Input: part model. Units: mm. Frame: model coordinates. A direction names the side the tool comes from. Give positions to 0.01 mm unless a question says otherwise; leave off trailing zeros. Loops run counter-clockwise (first coordinate to the right, second up) from the corner with the lowest first, then second, coordinate; pieces in that order, holes last. Notation, with made-up numbers: M 15.5,-32.75 L 25.5,-32.75 A8 cw 25.5,-19.75 Z; hole C 32,35.5 d1. An arc over 180 degrees is marked long. One line per item, written item: value. Start each with the question number.
(1) Ray query, line 1 along X through (y, z) = (2.5, 0.7); line 2 along X through (y, z) = (47.5, 2.05); line 3 along X through (y, z) = (31, 1.15). Return the intervals inside material, ascending. Write a range as from..to.
(2) Pull-direction query (X, two-part tool) for faces 6 (the flat face through (42, 30, 1)), 7 (the flat face through (50, 12, 1)), 8 (the flat face through (0, 13, 1)), 9 (the flat face through (25, 25, 3)); classes: released by +X, released by -X, zero draft, split by the parting line, or undercut.
(3) Section D-D on x = 38.5. Output: boundary loops of the cut face in (y, z).
(4) Section C-C on y = 2.5. Output: boundary loops of the cut face in (x, z).
(5) Section A-A on x = 25. Output: boundary loops of the cut face in (y, z).
(6) Access query for faces 1 (the flat face through (45, 37, 2)), 2 (the flat face through (25, 50, 1)), 3 (the flat face through (3, 25, 2)), 4 (the flat face through (38, 36.5, 1)), 5 (the flat face through (25, 25, 0)). Directions: +Z, -Z, +X, -X, +Y, -Y. A direction counts if a zero-diameter tool reaches every point of the face in a straight line with its end or side. Return the directions, or none.
(7) Pin query (flat end, axial travel): P1, Ø0.9, axis at x = 47, z = 1, coming from the +Y side; P2, Ø0.9, axis at y = 40, z = 1, coming from the -X side; P3, Ø1.5, axis at y = 29, z = 1.5, coming from the +X side. Return the tip coordinate at first contact, or that it passes through.
(8) Section B-B on z = 2.2. Output: boundary loops of the cut face in (x, y), plus the area to 3 significant figures.
Autodesk Inventor part; units mm, degrees
ref_plane "YZ Plane" through (0, 0, 0) normal (1, 0, 0) x (0, 1, 0)
ref_plane "XZ Plane" through (0, 0, 0) normal (0, 1, 0) x (-1, 0, 0)
ref_plane "XY Plane" through (0, 0, 0) normal (0, 0, 1) x (1, 0, 0)
sketch "Sketch1" plane through (0, 0, 0) normal (0, 0, 1) x (1, 0, 0)
  line L0 (0, 0) -> (50, 0)
  line L1 (50, 0) -> (50, 50)
  line L2 (50, 50) -> (0, 50)
  line L3 (0, 50) -> (0, 0)
  line L4 (25, 50) -> (25, 47.5)
  line L5 (0, 0) -> (5, 0)
  line L6 (5, 0) -> (5, 2.5)
  line L7 (50, 0) -> (45, 0)
  line L8 (45, 0) -> (45, 2.5)
  circle A0 centre (5, 2.5) radius 1.75
  circle A1 centre (45, 2.5) radius 1.75
  circle A2 centre (25, 47.5) radius 1.75
  line L9 (50, 50) -> (37, 50)
  line L10 (37, 50) -> (37, 30)
  line L11 (37, 30) -> (33, 30)
  line L12 (33, 30) -> (33, 23.5)
  line L13 (33, 23.5) -> (42, 23.5)
  line L14 (42, 23.5) -> (42, 36.5)
  line L15 (42, 36.5) -> (33, 36.5)
  line L16 (33, 36.5) -> (33, 30)
  dimension "d0" = 50
  dimension "d1" = 50
  dimension "d2" = 2.5
  dimension "d3" = 5
  dimension "d4" = 2.5
  dimension "d5" = 5
  dimension "d6" = 2.5
  dimension "d7" = 3.5
  dimension "d8" = 3.5
  dimension "d9" = 3.5
  dimension "d18" = 13
  dimension "d19" = 20
  dimension "d20" = 4
  dimension "d21" = 6.5
  dimension "d22" = 9
  dimension "d23" = 13
  dimension "d24" = 9
extrude "Extrusion1" add sketch "Sketch1" along normal blind 3
sketch "Sketch2" plane through (0, 0, 3) normal (0, 0, 1) x (1, 0, 0)
  line L0 (50, 50) -> (0, 50)
  line L1 (0, 50) -> (5, 50)
  line L2 (5, 50) -> (5, 25)
  line L3 (5, 25) -> (0, 25)
  line L4 (0, 50) -> (0, 0)
  line L5 (0, 25) -> (0, 50)
  line L6 (0, 50) -> (0, 25)
  line L7 (50, 0) -> (50, 50)
  line L8 (50, 50) -> (50, 25)
  line L9 (50, 25) -> (45, 25)
  line L10 (45, 25) -> (45, 50)
  line L11 (45, 50) -> (50, 50)
  dimension "d12" = 5
  dimension "d13" = 25
  dimension "d14" = 25
  dimension "d15" = 5
extrude "Extrusion2" cut sketch "Sketch2" against normal through all
properties part number "arm_0_bottom_case"
Output values:
1. line 1: x = 0..3.25, 6.75..43.25, 46.75..50
1. line 2: x = 5..23.25, 26.75..45
1. line 3: x = 5..33, 42..45
2. face 6: undercut
2. face 7: released by +X
2. face 8: released by -X
2. face 9: zero draft
3. outline: M 0,0 L 23.5,0 L 23.5,3 L 0,3 Z; M 36.5,0 L 50,0 L 50,3 L 36.5,3 Z
4. outline: M 0,0 L 3.25,0 L 3.25,3 L 0,3 Z; M 6.75,0 L 43.25,0 L 43.25,3 L 6.75,3 Z; M 46.75,0 L 50,0 L 50,3 L 46.75,3 Z
5. outline: M 0,0 L 45.75,0 L 45.75,3 L 0,3 Z; M 49.25,0 L 50,0 L 50,3 L 49.25,3 Z
6. face 1: +Z, -Z, +X, +Y
6. face 2: +Z, -Z, +X, -X, +Y
6. face 3: +Z, -Z, -X, +Y
6. face 4: +Z, -Z
6. face 5: -Z, +X, -X, +Y, -Y
7. P1: stops at y = 25
7. P2: stops at x = 5
7. P3: stops at x = 45
8. outline: M 0,0 L 50,0 L 50,25 L 45,25 L 45,50 L 5,50 L 5,25 L 0,25 Z; hole C 5,2.5 d3.5; hole C 25,47.5 d3.5; hole M 33,23.5 L 42,23.5 L 42,36.5 L 33,36.5 Z; hole C 45,2.5 d3.5
8. area: 2,100 mm²
